For this review, take the finished solid that the model builds, in its own axes (mm). A direction names the side the tool comes from. Round coordinates to 2 decimals unless told otherwise and drop trailing zeros. Order: outer loops, then holes, each group sorted by start corner. A loop starts at its lowest first (then second) coordinate and runs counter-clockwise, first axis right, second up. Notation, with made-up numbers: (-10.5, 45) - (13.5, 45) arc R22 ccw to (13.5, 70) - close; hole circle Ø10 at (4.5, -9.5). An arc over 180 degrees is marked (long way). One line per question, with ' | ' between items.
```python
from build123d import *

# Parameters (mm, degrees)
SKETCH1_W           = 21
SKETCH1_H           = 4
BOSS_EXTRUDE1_DEPTH = 15
BOSS_EXTRUDE2_DEPTH = 13
SKETCH3_R           = 1.8
CUT_EXTRUDE1_DEPTH  = 10
SKETCH4_W           = 9.565194399
SKETCH4_H           = 15
SKETCH4_R           = 1.8
SKETCH4_R_2         = 1.7
CUT_EXTRUDE2_DEPTH  = 15
SKETCH5_W           = 6
SKETCH5_H           = 10
CUT_EXTRUDE3_DEPTH  = 22
BOSS_EXTRUDE3_DEPTH = 54
SKETCH7_W           = 18
SKETCH7_H           = 15
CUT_EXTRUDE4_DEPTH  = 11


with BuildPart() as part:
    # Sketch1 → Boss-Extrude1 (new body)
    with BuildSketch(Plane.XY):
        Polygon((47, 0), (21, 0), (21, 26), (27, 26), (27, 4), (47, 4), align=None)
        with Locations((-10.5, 2)):
            Rectangle(SKETCH1_W, SKETCH1_H)
        with Locations((10.5, 2)):
            Rectangle(SKETCH1_W, SKETCH1_H)
        Polygon((-47, 0), (-21, 0), (-21, 26), (-27, 26), (-27, 4), (-47, 4), align=None)
    extrude(amount=BOSS_EXTRUDE1_DEPTH)

    # Sketch2 → Boss-Extrude2 (add)
    with BuildSketch(Plane(origin=(0, 0, 0), x_dir=(-1, 0, 0), z_dir=(0, 0, -1))):
        Polygon((-27, 26), (-27, 0), (27, 0), (27, 4), (27, 26), (21, 26), (21, 4), (-21, 4), (-21, 26), align=None)
    extrude(amount=BOSS_EXTRUDE2_DEPTH)

    # Sketch3 → Cut-Extrude1 (cut)
    with BuildSketch(Plane(origin=(0, 0, -13), x_dir=(-1, 0, 0), z_dir=(0, 0, -1))):
        with BuildLine():
            ThreePointArc((-22.2, 20.95), (-22.727207794, 22.222792206), (-24, 22.75))
            Line((-24, 22.75), (-24, 20.95))
            Line((-24, 20.95), (-24, 19.15))
            ThreePointArc((-24, 19.15), (-22.727207794, 19.677207794), (-22.2, 20.95))
        make_face()
        with BuildLine():
            Line((-24, 20.95), (-24, 22.75))
            ThreePointArc((-24, 22.75), (-25.8, 20.95), (-24, 19.15))
            Line((-24, 19.15), (-24, 20.95))
        make_face()
        with Locations((-24, 11.05)):
            Circle(SKETCH3_R)
        with Locations((24, 20.95)):
            Circle(SKETCH3_R)
        with Locations((24, 11.05)):
            Circle(SKETCH3_R)
    extrude(amount=-CUT_EXTRUDE1_DEPTH, mode=Mode.SUBTRACT)

    # Sketch4 → Cut-Extrude2 (cut)
    with BuildSketch(Plane(origin=(0, 4, 0), x_dir=(1, 0, 0), z_dir=(0, 1, 0))):
        with Locations((-42.2174028, -7.5)):
            Rectangle(SKETCH4_W, SKETCH4_H)
        with Locations(Location((-32.949794347, -7.5, 0), (0, 0, 180))):
            Circle(SKETCH4_R)
        with Locations(Location((42, -7.5, 0), (0, 0, 180))):
            Circle(SKETCH4_R_2)
        with Locations(Location((34, -7.5, 0), (0, 0, 180))):
            Circle(SKETCH4_R_2)
    extrude(amount=-CUT_EXTRUDE2_DEPTH, mode=Mode.SUBTRACT)

    # Sketch5 → Cut-Extrude3 (cut)
    with BuildSketch(Plane(origin=(0, 26, 0), x_dir=(1, 0, 0), z_dir=(0, 1, 0))):
        with Locations((-24, -10)):
            Rectangle(SKETCH5_W, SKETCH5_H)
    extrude(amount=-CUT_EXTRUDE3_DEPTH, mode=Mode.SUBTRACT)

    # Sketch6 → Boss-Extrude3 (add)
    with BuildSketch(Plane.ZY.offset(27)):
        Polygon((-13, 0), (0, 0), (0, -15), align=None)
    extrude(amount=-BOSS_EXTRUDE3_DEPTH)

    # Sketch7 → Cut-Extrude4 (cut)
    with BuildSketch(Plane(origin=(0, 0, -13), x_dir=(-1, 0, 0), z_dir=(0, 0, -1))):
        with Locations((-12, -7.5)):
            Rectangle(SKETCH7_W, SKETCH7_H)
        with Locations((12, -7.5)):
            Rectangle(SKETCH7_W, SKETCH7_H)
    extrude(amount=-CUT_EXTRUDE4_DEPTH, mode=Mode.SUBTRACT)


solid = part.part
```
(1) Mouldability with a two-part tool opening along Y and no side actions: class faces 5 (the cylindrical face through (-25.663, 10.361, -8.07)), 6 (the flat face through (27, 10, 1)), 7 (the flat face through (12, 0, -8)) as released by +Y, released by -Y, zero draft, split by the parting line, or undercut.
Output values:
face 5: undercut | face 6: zero draft | face 7: released by -Y
(2) Insertion check: pin 1 (1 mm diameter, centred on x = 12, z = 4, fed in from +Y); pin 2 (3.5 mm diameter, centred on y = -5.5, z = -10, fed in from -X); pin 3 (4 mm diameter, centred on x = 23, y = 11.5, fed in from -Z); pin 4 (5 mm diameter, centred on x = 3, z = 4, fed in from -Y). Each pin has a flat end and moves straight along its axis. Give the tip position at first contact, or say it passes through.
Output values:
pin 1: y = 4 | pin 2: x = -27 | pin 3: z = -13 | pin 4: y = 0
(3) For faces 1 (the flat face through (-12, -6, -2)), 2 (the flat face through (-21, 15, -4)), 3 (the flat face through (24, 21, -3)), 4 (the flat face through (0, -7, 0)), list the 3-axis set-ups (+Z, -Z, +X, -X, +Y, -Y) from which the entire face can be reached by the end or side of a thin tool; tool diameter is ignored.
Output values:
face 1: -Z, -Y | face 2: +Z, -Z, +Y | face 3: -Z | face 4: +Z, +X, -X, -Y
(4) We need section B-B on x = 42. State the section outline as (y, z) points, plus the area to 3 significant figures.
Output values:
outline: (0, 0) - (4, 0) - (4, 5.8) - (0, 5.8) - close; (0, 9.2) - (4, 9.2) - (4, 15) - (0, 15) - close | area: 46.4 mm^2
(5) We need section A-A on y = 1. State the section outline as (x, z) points, plus the area to 3 significant figures.
Output values:
outline: (-37.43, 0) - (-27, 0) - (-27, -13) - (27, -13) - (27, 0) - (47, 0) - (47, 15) - (-37.43, 15) - close; hole circle Ø3.6 at (-32.95, 7.5); hole circle Ø3.4 at (34, 7.5); hole circle Ø3.4 at (42, 7.5) | area: 1,940 mm^2
(6) We need section D-D on z = -4.5. State the section outline as (x, y) points.
Output values:
outline: (-27, -9.81) - (-21, -9.81) - (-21, 0) - (-3, 0) - (-3, -9.81) - (3, -9.81) - (3, 0) - (21, 0) - (21, -9.81) - (27, -9.81) - (27, 26) - (21, 26) - (21, 4) - (-21, 4) - (-21, 26) - (-27, 26) - close; hole circle Ø3.6 at (-24, 11.05); hole circle Ø3.6 at (-24, 20.95); hole circle Ø3.6 at (24, 11.05); hole circle Ø3.6 at (24, 20.95)
(7) For probe 1 along Y at (x, z) = (-24, -8.75); probe 2 along Z at (x, y) = (34, 1); probe 3 along X at (y, z) = (7, -8.5), list the stretches that pass through material, from the lowest coordinate up. Write a range as [from, to].
Output values:
probe 1: [-4.9, 9.25], [12.85, 19.15], [22.75, 26] | probe 2: [0, 5.8], [9.2, 15] | probe 3: [-27, -21], [21, 27]
(8) We need section C-C on y = 15.5. State the section outline as (x, z) points.
Output values:
outline: (-27, -13) - (-21, -13) - (-21, 5) - (-27, 5) - close; (21, -13) - (27, -13) - (27, 15) - (21, 15) - close
